Here's how the part is built. I have some questions about the finished solid (model axes, mm). A direction names the side the tool comes from. Coordinates: 2 decimals unless noted, no trailing zeros. Write each loop counter-clockwise with the first axis right and the second up, starting at its lowest first coordinate (ties: lowest second). Pieces come first, ordered by that corner, then holes.
Item 1: If we mould it in two halves opening along Y, with no side actions, what happens to faces 1 (the face through (5.5, -0.2, 0.1)), 2 (the face through (4, -1.206, 0)), 3 (the face through (10, 1.391, 0)), 4 (the face through (15, 3.969, -5))? For each: pulls with the +Y half, pulls with the -Y half, needs draft (parallel to the pull), parting line crosses it, or undercut.
Item 2: Please list where these lines run through material, in increasing order: line 1 (Y direction, x = 21, z = -30); line 2 (Z direction, x = 41.5, y = 1.15); line 3 (X direction, y = 1.3, z = 0).
Item 3: I'm going to push flat-ended pins straight in: P1, Ø2, axis at x = 31.5, y = 0, coming from the -Z side; P2, Ø1, axis at y = 1.5, z = 13.5, coming from the +X side; P3, Ø1, axis at y = 1, z = -26.5, coming from the -X side. Where does each tip first touch, or does it pass through?
Item 4: For faces 5 (the face through (-3, 1, 3.5)), 6 (the face through (9.8, 2.4, 2.5)), 7 (the face through (-2, 0, -5.5)), 8 (the face through (27.886, 2.359, -20.899)), 9 (the face through (-2, 0, 5.5)), which set-ups out of +Z, -Z, +X, -X, +Y, -Y let a thin tool reach every point of the face, with its end or its side?
Item 5: I want a section at D-D (z = -8). Please give me the cut outline in (x, y).
Item 6: I want a section at A-A (z = 0). Please give me the cut outline in (x, y), and give its area (3 significant figures).
Item 7: I want a section at C-C (x = 21). Please give me the cut outline in (y, z), and give its area (3 significant figures).
from build123d import *

# Parameters (mm, degrees)
BOSS_EXTRUDE1_DEPTH = 4.7625
SKETCH5_R           = 3.5000057
CUT_EXTRUDE2_DEPTH  = 3.37125
CUT_EXTRUDE3_DEPTH  = 1.98
SKETCH10_W          = 6.35
SKETCH10_H          = 0.79375
SKETCH10_W_2        = 35.745198541
SKETCH10_W_3        = 19.548012242
CUT_EXTRUDE4_DEPTH  = 63.97959256
CUT_EXTRUDE5_DEPTH  = 2.54
BOSS_EXTRUDE2_DEPTH = 2


with BuildPart() as part:
    # Sketch1 → Boss-Extrude1 (new body)
    with BuildSketch(Plane(origin=(0, 0, 0), x_dir=(1, 0, 0), z_dir=(0, 1, 0))):
        with BuildLine():
            ThreePointArc((47.438128512, -23.001108739), (21.083895316, -12.623567162), (23.295952901, 15.613744639))
            Line((23.295952901, 15.613744639), (32.606191406, 26.334377035))
            ThreePointArc((32.606191406, 26.334377035), (32.033289602, 35.241600739), (23.119772343, 34.776777479))
            Line((23.119772343, 34.776777479), (-4.692006503, 4.278735207))
            ThreePointArc((-4.692006503, 4.278735207), (-6.274930424, -0.973523588), (-3.175, -5.499261314))
            Line((-3.175, -5.499261314), (27.78125, -23.371860585))
            ThreePointArc((27.78125, -23.371860585), (37.752424387, -26.756618196), (48.25987898, -26.067923237))
            ThreePointArc((48.25987898, -26.067923237), (49.382410995, -24.123640754), (47.438128512, -23.001108739))
        make_face()
    extrude(amount=BOSS_EXTRUDE1_DEPTH)

    # Sketch5 → Cut-Extrude2 (cut)
    with BuildSketch(Plane.XZ):
        Circle(SKETCH5_R)
        with BuildLine():
            ThreePointArc((0, -3.5000057), (-3.5000057, 0), (0, 3.5000057))
            Line((0, 3.5000057), (-5.298345034, 3.5000057))
            ThreePointArc((-5.298345034, 3.5000057), (-6.35, 0), (-5.298345034, -3.5000057))
            Line((-5.298345034, -3.5000057), (0, -3.5000057))
        make_face()
    extrude(amount=-CUT_EXTRUDE2_DEPTH, mode=Mode.SUBTRACT)

    # Sketch6 → Cut-Extrude3 (cut)
    with BuildSketch(Plane.XZ.offset(-3.37125)):
        with BuildLine():
            Line((17.802786704, -2), (17.802786704, 2))
            Line((17.802786704, 2), (1.802786704, 3))
            ThreePointArc((1.802786704, 3), (3.5000057, 0), (1.802786704, -3))
            Line((1.802786704, -3), (17.802786704, -2))
        make_face()
    extrude(amount=CUT_EXTRUDE3_DEPTH, mode=Mode.SUBTRACT)

    # Sketch10 → Cut-Extrude4 (cut, through all)
    with BuildSketch(Plane(origin=(-3.175, 0, 5.499261314), x_dir=(0.866025404, 0, 0.5), z_dir=(-0.5, 0, 0.866025404))):
        with Locations((-3.175, 4.365625)):
            Rectangle(SKETCH10_W, SKETCH10_H)
        with Locations((17.872599271, 4.365625)):
            Rectangle(SKETCH10_W_2, SKETCH10_H)
        with Locations((45.519204662, 4.365625)):
            Rectangle(SKETCH10_W_3, SKETCH10_H)
        with Locations((45.519204662, 0.396875)):
            Rectangle(SKETCH10_W_3, SKETCH10_H)
        with Locations((17.872599271, 0.396875)):
            Rectangle(SKETCH10_W_2, SKETCH10_H)
        with Locations((-3.175, 0.396875)):
            Rectangle(SKETCH10_W, SKETCH10_H)
    extrude(amount=-CUT_EXTRUDE4_DEPTH, mode=Mode.SUBTRACT)

    # Sketch11 → Cut-Extrude5 (cut)
    with BuildSketch(Plane.XZ.offset(-3.37125)):
        with BuildLine():
            Line((-5.298345034, 3.5000057), (0, 3.5000057))
            ThreePointArc((0, 3.5000057), (3.5000057, 0), (0, -3.5000057))
            Line((0, -3.5000057), (-5.298345034, -3.5000057))
            ThreePointArc((-5.298345034, -3.5000057), (-6.35, 0), (-5.298345034, 3.5000057))
        make_face()
    extrude(amount=-CUT_EXTRUDE5_DEPTH, mode=Mode.SUBTRACT)

    # Sketch12 → Boss-Extrude2 (add)
    with BuildSketch(Plane.XZ.offset(-0.79375)):
        with BuildLine():
            Line((-3.175, 5.499261314), (-3.173710686, 5.5000057))
            Line((-3.173710686, 5.5000057), (0, 5.5000057))
            ThreePointArc((0, 5.5000057), (5.5000057, 0), (0, -5.5000057))
            Line((0, -5.5000057), (-3.57830535, -5.5000057))
            Line((-3.57830535, -5.5000057), (-4.692006503, -4.278735207))
            ThreePointArc((-4.692006503, -4.278735207), (-5.010327921, -3.901168303), (-5.298345034, -3.5000057))
            Line((-5.298345034, -3.5000057), (0, -3.5000057))
            ThreePointArc((0, -3.5000057), (3.5000057, 0), (0, 3.5000057))
            Line((0, 3.5000057), (-5.298345034, 3.5000057))
            ThreePointArc((-5.298345034, 3.5000057), (-4.353004683, 4.623186156), (-3.175, 5.499261314))
        make_face()
    extrude(amount=BOSS_EXTRUDE2_DEPTH)


solid = part.part
Answer:
1. face 1: needs draft
1. face 2: pulls with the -Y half
1. face 3: undercut
1. face 4: pulls with the +Y half
2. line 1: y = 0.79 to 3.97
2. line 2: z = 23.81 to 26.99
2. line 3: x = 3.5 to 17.46
3. P1: stops at z = -36.05
3. P2: stops at x = 22.01
3. P3: stops at x = 15.12
4. face 5: -X, +Y, -Y
4. face 6: -X
4. face 7: -Z, +X, -X, -Y
4. face 8: +X, +Y, -Y
4. face 9: +Z, +X, -X, -Y
5. outline: (-1.3, 0.79) - (18.85, 0.79) - (18.85, 3.97) - (-1.3, 3.97) - close
6. outline: (3.5, -1.21) - (5.5, -1.21) - (5.5, 0.79) - (17.46, 0.79) - (17.46, 1.39) - (3.5, 1.39) - close; (3.5, 3.37) - (17.46, 3.37) - (17.46, 3.97) - (3.5, 3.97) - close
6. area: 20.7 mm2
7. outline: (0.79, -32.45) - (3.97, -32.45) - (3.97, -12.49) - (0.79, -12.49) - close; (0.79, 12.49) - (3.97, 12.49) - (3.97, 19.46) - (0.79, 19.46) - close
7. area: 85.5 mm2
